from build123d import *

# Parameters (mm, degrees)
F1_DEPTH = 457.2
F2_R     = 4.7625
F3_DEPTH = 25.4


with BuildPart() as f1:
    # F0 (on Front) → F1 (new body)
    with BuildSketch(Plane.XZ):
        with BuildLine():
            Line((-8.715044, -12.260614), (10.334956, -12.260614))
            ThreePointArc((10.334956, -12.260614), (12.58002, -11.330678), (13.509956, -9.085614))
            Line((13.509956, -9.085614), (13.509956, 9.964386))
            ThreePointArc((13.509956, 9.964386), (12.58002, 12.20945), (10.334956, 13.139386))
            Line((10.334956, 13.139386), (-8.715044, 13.139386))
            ThreePointArc((-8.715044, 13.139386), (-10.960108, 12.20945), (-11.890044, 9.964386))
            Line((-11.890044, 9.964386), (-11.890044, -9.085614))
            ThreePointArc((-11.890044, -9.085614), (-10.960108, -11.330678), (-8.715044, -12.260614))
        make_face()
        with BuildLine():
            ThreePointArc((10.334956, -5.910614), (9.40502, -8.155678), (7.159956, -9.085614))
            Line((7.159956, -9.085614), (-5.540044, -9.085614))
            ThreePointArc((-5.540044, -9.085614), (-7.785108, -8.155678), (-8.715044, -5.910614))
            Line((-8.715044, -5.910614), (-8.715044, 6.789386))
            ThreePointArc((-8.715044, 6.789386), (-7.785108, 9.03445), (-5.540044, 9.964386))
            Line((-5.540044, 9.964386), (7.159956, 9.964386))
            ThreePointArc((7.159956, 9.964386), (9.40502, 9.03445), (10.334956, 6.789386))
            Line((10.334956, 6.789386), (10.334956, -5.910614))
        make_face(mode=Mode.SUBTRACT)
    extrude(amount=F1_DEPTH)

    # F2 (on face) → F3 (cut)
    with BuildSketch(Plane.XY.offset(13.139386)):
        with Locations((0, -11.1125)):
            Circle(F2_R)
    extrude(amount=-F3_DEPTH, mode=Mode.SUBTRACT)


solid = f1.part
Input: part model. Units: mm. Frame: model coordinates. A direction names the side the tool comes from. Coordinates: 2 decimals unless noted, no trailing zeros. Loops run counter-clockwise (first coordinate to the right, second up) from the corner with the lowest first, then second, coordinate; pieces in that order, holes last. Notation, with made-up numbers: (1, 63.5) -> (56, 63.5) arc R27 cw to (56, 86.5) -> close; hole circle Ø9 at (-16.75, 73). An arc over 180 degrees is marked (long way). Write each question's results on one line, items separated by ' | '. Start each with the question number.
Q1. Section B-B, the plane y = -320.5. Return the cut outline in (x, z) (3 decimals), plus the area to 3 significant figures.
Q2. Reachability of faces 4 (the flat face through (-11.89, -225, 1)), 5 (the flat face through (1, -225, 9.964)) from +Z, -Z, +X, -X, +Y, -Y: full face, straight path, thin tool, end or side. Return the list, or none.
Q3. Section A-A, the plane z = -1.5. Return the cut outline in (x, y).
Q4. Pull-direction query (Z, two-part tool) for faces 1 (the flat face through (-11, -457.2, 1)), 2 (the flat face through (1, -225, -12.261)), 3 (the flat face through (1, -225, -9.086)); classes: released by +Z, released by -Z, zero draft, split by the parting line, or undercut.
Q5. Ray query, line 1 (Z direction, x = 3.75, y = -391); line 2 (Y direction, x = 0, z = 12.45) (3 decimals); line 3 (X direction, y = -346, z = 1.75). Return the intervals inside material, ascending. Write a range as from..to.
Q6. Section C-C, the plane x = 0. Return the cut outline in (y, z) (3 decimals).
Found:
1) outline: (-11.89, -9.086) arc R3.175 ccw to (-8.715, -12.261) -> (10.335, -12.261) arc R3.175 ccw to (13.51, -9.086) -> (13.51, 9.964) arc R3.175 ccw to (10.335, 13.139) -> (-8.715, 13.139) arc R3.175 ccw to (-11.89, 9.964) -> close; hole (-8.715, -5.911) arc R3.175 ccw to (-5.54, -9.086) -> (7.16, -9.086) arc R3.175 ccw to (10.335, -5.911) -> (10.335, 6.789) arc R3.175 ccw to (7.16, 9.964) -> (-5.54, 9.964) arc R3.175 ccw to (-8.715, 6.789) -> close | area: 282 mm2
2) face 4: +Z, -Z, -X, +Y, -Y | face 5: +Y, -Y
3) outline: (-11.89, -457.2) -> (-8.72, -457.2) -> (-8.72, 0) -> (-11.89, 0) -> close; (10.33, -457.2) -> (13.51, -457.2) -> (13.51, 0) -> (10.33, 0) -> close
4) face 1: zero draft | face 2: released by -Z | face 3: undercut
5) line 1: -12.26..-9.09, 9.96..13.14 | line 2: -457.2..-15.875, -6.35..0 | line 3: -11.89..-8.72, 10.33..13.51
6) outline: (-457.2, -12.261) -> (-15.875, -12.261) -> (-15.875, -9.086) -> (-457.2, -9.086) -> close; (-457.2, 9.964) -> (-15.875, 9.964) -> (-15.875, 13.139) -> (-457.2, 13.139) -> close; (-6.35, -12.261) -> (0, -12.261) -> (0, -9.086) -> (-6.35, -9.086) -> close; (-6.35, 9.964) -> (0, 9.964) -> (0, 13.139) -> (-6.35, 13.139) -> close
